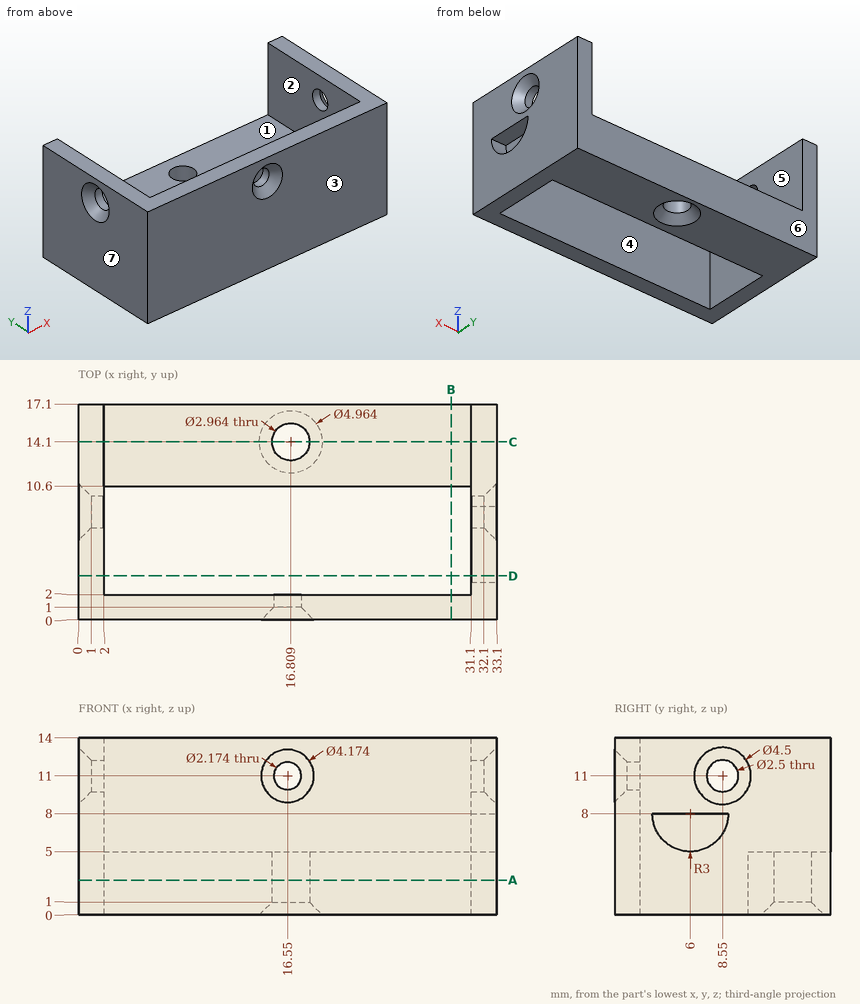
Design review of the part shown in the three views and the two pictorial views. Dimensions are in mm from the part's minimum x, y and z. A direction names the side the tool comes from. Give positions to 0.01 mm unless a question says otherwise; leave off trailing zeros. Order: outer loops, then holes, each group sorted by start corner. A loop starts at its lowest first (then second) coordinate and runs counter-clockwise, first axis right, second up. Notation, with made-up numbers: M 19.5,74 L 76.5,74 A11 ccw 76.5,84 Z; hole C 13,-24 d3. An arc over 180 degrees is marked long. Answer in a Markdown table with one row per item. Add a question column.
(1) Mouldability with a two-part tool opening along X and no side actions: class the marked faces 5, 6 and 7 as +X half, -X half, draft (parallel to the pull), parting line (faces both ways), or undercut.
(2) For pin 1 (3.5 mm diameter, centred on x = 16.81, y = 14.1, fed in from +Z); pin 2 (3 mm diameter, centred on y = 8.55, z = 11, fed in from -X); pin 3 (2 mm diameter, centred on y = 8.55, z = 11, fed in from +X); pin 4 (3 mm diameter, centred on x = 16.55, z = 11, fed in from -Y), all flat-tipped, find the tip position at first contact; note any pin that passes through.
(3) For the marked faces 1, 2, 3 and 4, list the 3-axis set-ups (+Z, -Z, +X, -X, +Y, -Y) from which the entire face can be reached by the end or side of a thin tool; tool diameter is ignored.
(4) Wall thickness on probe 1 along Y at (x, z) = (12, 3); probe 2 along X at (y, z) = (1.7, 11); probe 3 along X at (y, z) = (10, 2): over which ranges is each line inside the solid? List them lowest first. Write a range as [from, to].
(5) Consider section D-D on y = 3.5. State the section outline as (x, z) points.
(6) Consider section B-B on x = 29.5. State the section outline as (y, z) points.
(7) Consider section A-A on z = 2.75. State the section outline as (x, y) points.
(8) Consider section C-C on y = 14.1. State the section outline as (x, z) points.
Evaluation:
| question | item | result |
|---|---|---|
| 1 | face 5 | undercut |
| 1 | face 6 | draft |
| 1 | face 7 | -X half |
| 2 | pin 1 | stops at z = 5 |
| 2 | pin 2 | stops at x = 0.75 |
| 2 | pin 3 | passes through |
| 2 | pin 4 | stops at y = 0.59 |
| 3 | face 1 | +Z, +Y |
| 3 | face 2 | +Z |
| 3 | face 3 | +Z, -Z, +X, -X, -Y |
| 3 | face 4 | +Z, -Z |
| 4 | probe 1 | y = [0, 2], [10.6, 17.1] |
| 4 | probe 2 | x = [0, 15.46], [17.64, 33.1] |
| 4 | probe 3 | x = [0, 2], [31.1, 33.1] |
| 5 | outline | M 0,0 L 2,0 L 2,14 L 0,14 Z; M 31.1,0 L 33.1,0 L 33.1,6.34 L 31.1,6.34 Z; M 31.1,8 L 33.1,8 L 33.1,14 L 31.1,14 Z |
| 6 | outline | M 0,0 L 2,0 L 2,14 L 0,14 Z; M 10.6,0 L 17.1,0 L 17.1,5 L 10.6,5 Z |
| 7 | outline | M 0,0 L 33.1,0 L 33.1,17.1 L 0,17.1 Z; hole M 2,2 L 31.1,2 L 31.1,10.6 L 2,10.6 Z; hole C 16.81,14.1 d2.96 |
| 8 | outline | M 0,0 L 14.33,0 L 15.33,1 L 15.33,5 L 2,5 L 2,14 L 0,14 Z; M 18.29,1 L 19.29,0 L 33.1,0 L 33.1,14 L 31.1,14 L 31.1,5 L 18.29,5 Z |
